Geometry check sheet. Reference: drawing and pictorial views, mm from the part's lowest x, y, z. Give positions to 0.01 mm unless a question says otherwise; leave off trailing zeros. Write each loop counter-clockwise with the first axis right and the second up, starting at its lowest first coordinate (ties: lowest second). Pieces come first, ordered by that corner, then holes. Notation, with made-up numbers: (-31, -19.5) -> (-16, -19.5) arc R6 cw to (-16, -11.5) -> close; hole circle Ø7 at (27, 63.25). An arc over 180 degrees is marked (long way). Use a Markdown table: item, result. Add a question column.
1. Release check for a two-part mould opening along Y. For the marked faces 1, 2, 3 and 4 record: released by +Y, released by -Y, zero draft, split by the parting line, or undercut.
2. Cross-section at C-C (z = 0.65). Enter the section's corners in (x, y), then the cut area to 3 significant figures.
3. Cross-section at A-A (y = 10). Enter the section's corners in (x, z).
4. Gauge pin test, flat end, axial feed: P1, Ø2.5, axis at x = 20, y = 10, coming from the -Z side. Record the tip position at first contact, or that the pin passes through.
5. Scan lines: probe 1 along Y at (x, z) = (20, 2.75); probe 2 along X at (y, z) = (9, 3.85); probe 3 along X at (y, z) = (18.75, 1.05). Record each from-to range of solid material in increasing order. Write a range as [from, to].
6. Cross-section at B-B (x = 20). Enter the section's corners in (y, z), then the cut area to 3 significant figures.
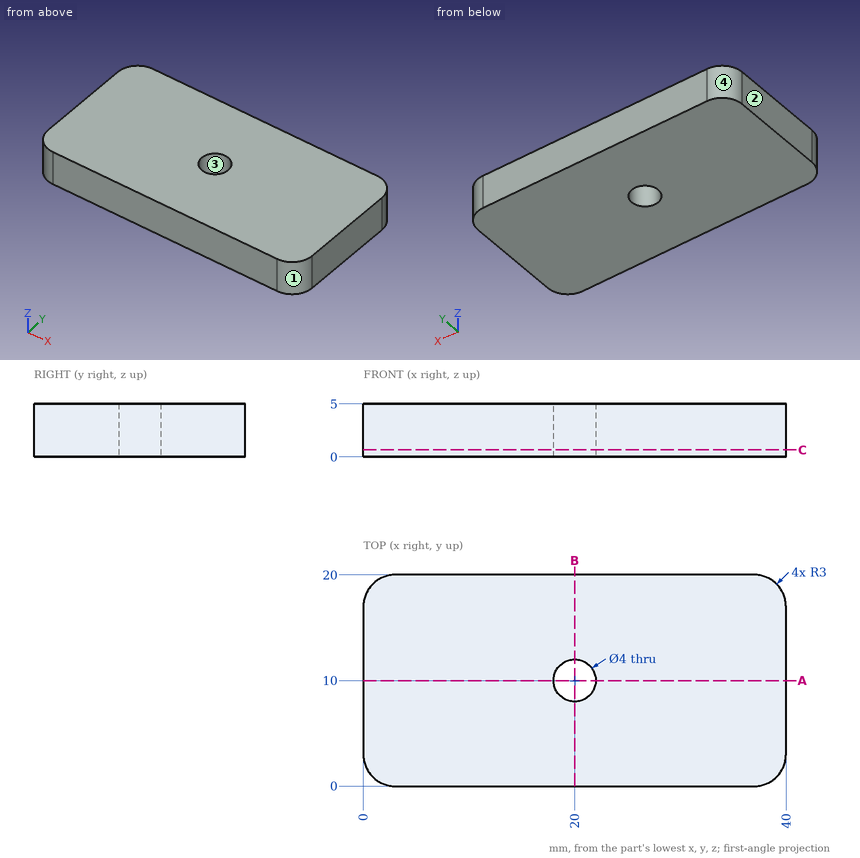
Worked answers:
| question | item | result |
|---|---|---|
| 1 | face 1 | released by -Y |
| 1 | face 2 | zero draft |
| 1 | face 3 | undercut |
| 1 | face 4 | released by +Y |
| 2 | outline | (0, 3) arc R3 ccw to (3, 0) -> (37, 0) arc R3 ccw to (40, 3) -> (40, 17) arc R3 ccw to (37, 20) -> (3, 20) arc R3 ccw to (0, 17) -> close; hole circle Ø4 at (20, 10) |
| 2 | area | 780 mm² |
| 3 | outline | (0, 0) -> (18, 0) -> (18, 5) -> (0, 5) -> close; (22, 0) -> (40, 0) -> (40, 5) -> (22, 5) -> close |
| 4 | P1 | passes through |
| 5 | probe 1 | y = [0, 8], [12, 20] |
| 5 | probe 2 | x = [0, 18.27], [21.73, 40] |
| 5 | probe 3 | x = [0.56, 39.44] |
| 6 | outline | (0, 0) -> (8, 0) -> (8, 5) -> (0, 5) -> close; (12, 0) -> (20, 0) -> (20, 5) -> (12, 5) -> close |
| 6 | area | 80.0 mm² |
